Autodesk Inventor part; units mm, degrees
ref_plane "Work Plane1" through (0, 0, -10) normal (0, 0, 1) x (1, 0, 0)
ref_plane "Work Plane3" through (0, 0, -38) normal (0, 0, 1) x (1, 0, 0)
ref_plane "YZ Plane" through (0, 0, 0) normal (1, 0, 0) x (0, 1, 0)
sketch "Sketch1" plane through (0, 0, 0) normal (0, 0, 1) x (1, 0, 0)
  circle A0 centre (0, 0) radius 12.5
  circle A1 centre (0, 0) radius 9
  circle A2 centre (0, 0) radius 11
  line L0 (17, -21) -> (-17, -21)
  line L1 (-21, -17) -> (-21, 17)
  line L2 (-17, 21) -> (17, 21)
  line L3 (21, 17) -> (21, -17)
  line L4 (21, -21) -> (-21, 21) construction
  line L5 (-21, -21) -> (21, 21) construction
  arc A3 (-17, 21) -> (-21, 17) centre (-17, 17) ccw
  arc A4 (-21, -17) -> (-17, -21) centre (-17, -17) ccw
  arc A5 (17, -21) -> (21, -17) centre (17, -17) ccw
  arc A6 (21, 17) -> (17, 21) centre (17, 17) ccw
  line L6 (15.5, -15.5) -> (-15.5, -15.5) construction
  line L7 (-15.5, -15.5) -> (-15.5, 15.5) construction
  line L8 (-15.5, 15.5) -> (15.5, 15.5) construction
  line L9 (15.5, 15.5) -> (15.5, -15.5) construction
  line L10 (15.5, -15.5) -> (-15.5, 15.5) construction
  line L11 (-15.5, -15.5) -> (15.5, 15.5) construction
  circle A7 centre (0, 0) radius 2.5
  circle A8 centre (0, 0) radius 4
  dimension "d0" = 42
  dimension "d2" = 42
  dimension "d3" = 4
  dimension "d4" = 18
  dimension "d5" = 22
  dimension "d6" = 25
  dimension "d7" = 31
  dimension "d22" = 5
  dimension "d23" = 8
ref_plane "Work Plane1" through (0, 0, -10) normal (0, 0, 1) x (1, 0, 0)
ref_plane "Work Plane3" through (0, 0, -38) normal (0, 0, 1) x (1, 0, 0)
ref_plane "Work Plane2" through (0, 0, -48) normal (0, 0, 1) x (1, 0, 0)
extrude "Extrusion1" add sketch "Sketch1" against normal up to surface (10 mm away) from surface at 0 contours A0 | A1 | A2 | L0 A4 L1 A3 L2 A6 L3 A5 | A7 | A8
sketch "Sketch2" plane through (17, 21, -10) normal (0, 0, -1) x (-1, 0, 0)
  arc A0 (34, -42) -> (38, -38) centre (34, -38) ccw
  line L0 (38, -38) -> (38, -4)
  arc A1 (38, -4) -> (34, 0) centre (34, -4) ccw
  line L1 (34, 0) -> (0, 0)
  arc A2 (0, 0) -> (-4, -4) centre (0, -4) ccw
  line L2 (-4, -4) -> (-4, -38)
  arc A3 (-4, -38) -> (0, -42) centre (0, -38) ccw
  line L3 (0, -42) -> (34, -42)
  line L4 (0, -0.1) -> (34, -0.1)
  arc A4 (37.9, -4) -> (34, -0.1) centre (34, -4) ccw
  line L5 (37.9, -4) -> (37.9, -38)
  arc A5 (34, -41.9) -> (37.9, -38) centre (34, -38) ccw
  line L6 (34, -41.9) -> (0, -41.9)
  arc A6 (-3.9, -38) -> (0, -41.9) centre (0, -38) ccw
  line L7 (-3.9, -38) -> (-3.9, -4)
  arc A7 (0, -0.1) -> (-3.9, -4) centre (0, -4) ccw
  point P0 (17, -21)
  dimension "d13" = 0.1
extrude "Extrusion2" add sketch "Sketch2" along normal up to surface (10 mm away) from surface at 28 contours L3 A3 L2 A2 L1 A1 L0 A0 | L4 A4 L5 A5 L6 A6 L7 A7
extrude "Extrusion3" add sketch "Sketch2" along normal up to surface (28 mm away) from surface at 0 contours L4 A4 L5 A5 L6 A6 L7 A7
extrude "Extrusion4" cut sketch "Sketch1" against normal blind 0.5 contours A0 | A1 | A8
extrude "Extrusion5" add sketch "Sketch1" along normal blind 2 contours A2
extrude "Extrusion6" cut sketch "Sketch1" against normal blind 2 contours A8
extrude "Extrusion7" add sketch "Sketch1" along normal blind 25 contours A7
hole "Hole1" at (-17, 17, 0) at (-17, -17, 0) at (17, -17, 0) at (17, 17, 0) direction (0, 0, -1) diameter 2.459 depth 4 tip angle 118
properties part number "nema17 48mm"
Here's how the part is built. I have some questions about the finished solid (model axes, mm). A direction names the side the tool comes from. Give positions to 0.01 mm unless a question says otherwise; leave off trailing zeros. Loops run counter-clockwise (first coordinate to the right, second up) from the corner with the lowest first, then second, coordinate; pieces in that order, holes last. Notation, with made-up numbers: (79, 22) -> (134, 22) arc R26 ccw to (134, 38) -> close; hole circle Ø9 at (74.5, 33.5). An arc over 180 degrees is marked (long way). Answer as a JSON object with one key per item and string values. Group by question number.
Item 1: Imagine slicing it at C-C on z = -23. Write out the boundary of the cut face in (x, y), then the cut area to 3 significant figures.
Item 2: On a 3-axis mill with a long thin cutter (end or side, diameter ignored), from which of +Z, -Z, +X, -X, +Y, -Y can I reach the whole of each face in a straight line? I mean faces 1 (the cylindrical face through (-1.172, -8.923, 0.732)), 2 (the flat face through (0, 20.9, -24)), 3 (the cylindrical face through (19.788, 19.727, -23.804)), 4 (the flat face through (20.9, 0, -24)). Say none if no direction works.
Item 3: I need wall thicknesses on L1, parallel to X at y = 17, z = -2; L2, parallel to Y at x = 0, z = 1.05. Which ranges of each line are inside material? Lowest first, please.
Item 4: Will these pins go through, and if not, where does the flat tip stop? pin 1 (22.5 mm diameter, centred on y = 4, z = -21.5, fed in from -X); pin 2 (1 mm diameter, centred on x = 4, z = -16.5, fed in from +Y); pin 3 (4 mm diameter, centred on x = -17, y = -17, fed in from +Z).
Item 5: Imagine slicing it at A-A on x = -14.5. Write out the boundary of the cut face in (y, z).
Item 6: Thinking about a two-plate mould opening in X: for faces 5 (the cylindrical face through (-19.797, 19.859, -4.93)), 6 (the cylindrical face through (19.797, -19.859, -4.93)), 7 (the cylindrical face through (-17.369, 15.827, -2.028)), which applies, pulls with the +X half, pulls with the -X half, needs draft (parallel to the pull), parting line crosses it, or undercut?
Answer list:
{
 "1": {"outline": "(-20.9, -17) arc R3.9 ccw to (-17, -20.9) -> (17, -20.9) arc R3.9 ccw to (20.9, -17) -> (20.9, 17) arc R3.9 ccw to (17, 20.9) -> (-17, 20.9) arc R3.9 ccw to (-20.9, 17) -> close", "area": "1,730 mm2"},
 "2": {"face 1": "+Z", "face 2": "+X, -X, +Y", "face 3": "+X, +Y", "face 4": "+X, +Y, -Y"},
 "3": {"L1": "x = -21 to -18.23, -15.77 to 15.77, 18.23 to 21", "L2": "y = -11 to -9, -2.5 to 2.5, 9 to 11"},
 "4": {"pin 1": "stops at x = -20.9", "pin 2": "stops at y = 20.9", "pin 3": "stops at z = 0"},
 "5": {"outline": "(-21, -48) -> (21, -48) -> (21, -38) -> (20.9, -38) -> (20.9, -10) -> (21, -10) -> (21, 0) -> (-21, 0) -> (-21, -10) -> (-20.9, -10) -> (-20.9, -38) -> (-21, -38) -> close"},
 "6": {"face 5": "pulls with the -X half", "face 6": "pulls with the +X half", "face 7": "undercut"}
}
